Part model, mm, in its own coordinate system. Give positions to 0.01 mm unless a question says otherwise; leave off trailing zeros. Loops run counter-clockwise (first coordinate to the right, second up) from the corner with the lowest first, then second, coordinate; pieces in that order, holes last. Notation, with made-up numbers: M 15.25,-36.75 L 63.25,-36.75 A17 cw 63.25,-3.75 Z; hole C 39,17.5 d5. An arc over 180 degrees is marked long. Put each result on its own line as item: value. Start each with the question number.
Autodesk Inventor part; units mm, degrees
ref_plane "YZ Plane" through (0, 0, 0) normal (1, 0, 0) x (0, 1, 0)
ref_plane "XZ Plane" through (0, 0, 0) normal (0, 1, 0) x (-1, 0, 0)
ref_plane "XY Plane" through (0, 0, 0) normal (0, 0, 1) x (1, 0, 0)
sketch "スケッチ1" plane through (0, 0, 0) normal (0, 0, 1) x (1, 0, 0)
  line L0 (203.1661, 661.0271) -> (203.1661, -646.9853)
  line L1 (203.1661, 628.7976) -> (183.1661, 628.7976)
  line L2 (183.1661, 660.9684) -> (183.1661, -646.9853)
  line L3 (183.1661, 25.0147) -> (203.1661, 25.0147)
  line L4 (183.1661, -646.9853) -> (203.1661, -646.9853)
  line L5 (183.1661, 660.9684) -> (203.1661, 661.0271)
  line L6 (168.1661, 612.8976) -> (195.9661, 612.8976)
  line L7 (195.9661, 612.8976) -> (195.9661, 628.7976)
  line L8 (195.9661, 628.7976) -> (168.1661, 628.7976)
  line L9 (168.1661, 628.7976) -> (168.1661, 612.8976)
  circle A0 centre (170.9661, 615.6976) radius 1.5
  circle A1 centre (193.1661, 625.9976) radius 1.5
  circle A2 centre (193.1661, 633.9976) radius 1.5
  line L10 (154.6661, 79.2604) -> (182.4661, 79.2604)
  line L11 (182.4661, 79.2604) -> (182.4661, 63.3604)
  line L12 (182.4661, 63.3604) -> (154.6661, 63.3604)
  line L13 (154.6661, 63.3604) -> (154.6661, 79.2604)
  circle A3 centre (157.4661, 76.4604) radius 1.5
  circle A4 centre (179.6661, 66.1604) radius 1.5
  circle A5 centre (193.1661, 64.3604) radius 1.5
  line L14 (183.1661, 638.9976) -> (203.1661, 638.9976)
  line L15 (195.9661, 612.8976) -> (203.1661, 612.8976)
  line L16 (203.1661, 612.8976) -> (203.1661, 638.9976)
  line L17 (183.1661, 638.9976) -> (168.1661, 628.7976)
  line L18 (183.1661, 59.3604) -> (203.1661, 59.3604)
  line L19 (182.4661, 79.2604) -> (203.1661, 79.2604)
  line L20 (203.1661, 79.2604) -> (203.1661, 59.3604)
  line L21 (183.1661, 59.3604) -> (154.6661, 63.3604)
  circle A6 centre (193.1661, 72.3604) radius 1.5
  point P0 (0, 0)
  point P1 (-212.8828, -214.6519)
  dimension "d0" = 672
  dimension "d1" = 27.8
  dimension "d2" = 15.9
  dimension "d3" = 3
  dimension "d4" = 3
  dimension "d5" = 2.8
  dimension "d6" = 2.8
  dimension "d7" = 2.8
  dimension "d8" = 2.8
  dimension "d9" = 0
  dimension "d10" = 10
  dimension "d11" = 3
  dimension "d12" = 8
  dimension "d13" = 10
  dimension "d14" = 27
  dimension "d15" = 27.8
  dimension "d16" = 15.9
  dimension "d17" = 3
  dimension "d18" = 3
  dimension "d19" = 2.8
  dimension "d20" = 2.8
  dimension "d21" = 2.8
  dimension "d22" = 2.8
  dimension "d24" = 560
  dimension "d25" = 3
  dimension "d27" = 10
  dimension "d28" = 5
  dimension "d29" = 5
  dimension "d33" = 20
  dimension "d34" = 203.1661
  dimension "d39" = 3.5
  dimension "d40" = 3
  dimension "d41" = 10
  dimension "d42" = 8
  dimension "d43" = 4
extrude "押し出し1" add sketch "スケッチ1" against normal blind 2 contours L0 L18 L2 L19 | L2 L21 L12 L11 L19 | L11 L12 L13 L10
fillet "フィレット1" radius 2 5 edges at (154.6661, 79.2604, -1) (154.6661, 63.3604, -1) (183.1661, 59.3604, -1) (203.1661, 59.3604, -1) (203.1661, 79.2604, -1)
equation "\"d6\" = d5"
equation "\"d7\" = d5"
equation "\"d8\" = d5"
equation "\"d20\" = d19"
equation "\"d21\" = d19"
equation "\"d22\" = d19"
properties part number "dribl-v1-Plate-12" material "アルミニウム 6061"
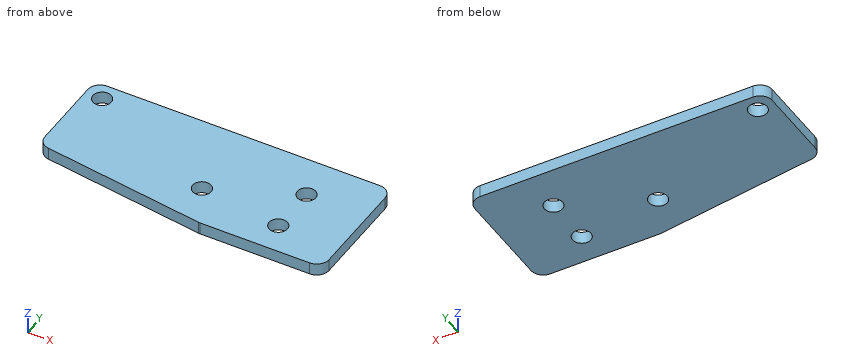
1) Wall check: L1, parallel to X at y = 76.5, z = -0.1; L2, parallel to X at y = 73.5, z = -1.75; L3, parallel to Y at x = 180, z = -1.35. Give the ranges that are in metal, low to high.
2) Band-saw the part on C-C on x = 158.5. Give the cut face in (y, z).
3) Band-saw the part on A-A on y = 71.75. Give the cut face in (x, z), then the cut area to 3 significant figures.
4) Band-saw the part on D-D on x = 171. Give the cut face in (y, z), then the cut area to 3 significant figures.
5) Band-saw the part on B-B on z = -1.2. Give the cut face in (x, y).
6) Pin check, flat tip, straight feed: pin 1 Ø1.8 at (x, y) = (193.17, 72.36) entering from +Z. Stop position of the tip, or through.
Evaluation:
1. L1: 154.67 to 155.97, 158.97 to 203.17
1. L2: 154.67 to 192.19, 194.14 to 203.17
1. L3: 59.8 to 64.7, 67.62 to 79.26
2. outline: M 62.82,-2 L 75.37,-2 L 75.37,0 L 62.82,0 Z; M 77.55,-2 L 79.26,-2 L 79.26,0 L 77.55,0 Z
3. outline: M 154.67,-2 L 191.8,-2 L 191.8,0 L 154.67,0 Z; M 194.54,-2 L 203.17,-2 L 203.17,0 L 194.54,0 Z
3. area: 91.5 mm2
4. outline: M 61.07,-2 L 79.26,-2 L 79.26,0 L 61.07,0 Z
4. area: 36.4 mm2
5. outline: M 154.67,65.1 A2 ccw 156.39,63.12 L 183.03,59.38 A2 ccw 183.31,59.36 L 201.17,59.36 A2 ccw 203.17,61.36 L 203.17,77.26 A2 ccw 201.17,79.26 L 156.67,79.26 A2 ccw 154.67,77.26 Z; hole C 157.47,76.46 d3; hole C 179.67,66.16 d3; hole C 193.17,64.36 d3; hole C 193.17,72.36 d3
6. pin 1: through
